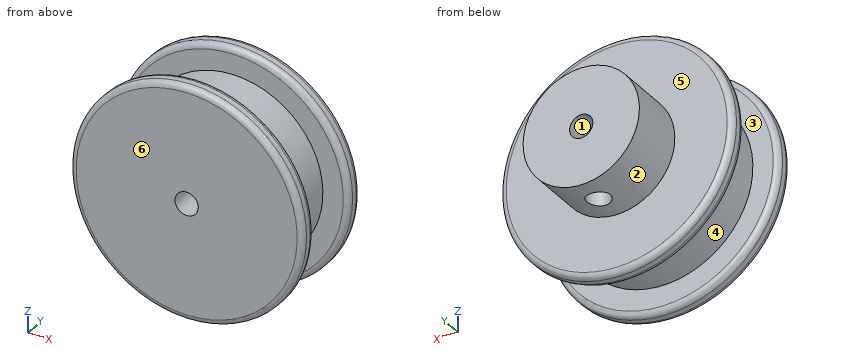
```python
from build123d import *

# Parameters (mm, degrees)
SKETCH_1_R          = 15.5
EXTRUDE_1_DEPTH     = 10
SKETCH_2_R          = 20
EXTRUDE_2_DEPTH     = 3
EXTRUDE_START       = 3
SKETCH_3_R          = 20
EXTRUDE_3_DEPTH     = 3
FILLET_2_R          = 1
SKETCH_4_R          = 2
CUT_EXTRUDE_1_DEPTH = 33.49615368
EXTRUDE_START_2     = 10
SKETCH_5_R          = 10
SKETCH_5_R_2        = 2
EXTRUDE_4_DEPTH     = 10
SKETCH_6_R          = 2
CUT_EXTRUDE_2_DEPTH = 37.455452322


with BuildPart() as part:
    # 草图1 → 凸台-拉伸1 (new body)
    with BuildSketch(Plane(origin=(0, 0, 0), x_dir=(1, 0, 0), z_dir=(0, 1, 0))):
        with Locations(Location((0, 0, 0), (0, 0, 270))):
            Circle(SKETCH_1_R)
    extrude(amount=EXTRUDE_1_DEPTH)

    # 草图2 → 凸台-拉伸2 (add)
    with BuildSketch(Plane(origin=(0, 10, 0), x_dir=(1, 0, 0), z_dir=(0, 1, 0))):
        with Locations(Location((0, 0, 0), (0, 0, 270))):
            Circle(SKETCH_2_R)
    extrude(amount=EXTRUDE_2_DEPTH)

    # 草图3 → 凸台-拉伸3 (add)
    with BuildSketch(Plane.XZ.offset(EXTRUDE_START)):
        with Locations(Location((0, 0, 0), (0, 0, 90))):
            Circle(SKETCH_3_R)
    extrude(amount=-EXTRUDE_3_DEPTH)

    # 圆角2
    fillet_2_edges = [part.edges().sort_by_distance(p)[0] for p in [
        (0, -3, -20),
        (0, 10, -20),
        (0, 13, -20),
        (0, 0, -20),
    ]]
    fillet(fillet_2_edges, radius=FILLET_2_R)

    # 草图4 → 切除-拉伸1 (cut, through all)
    with BuildSketch(Plane(origin=(0, 13, 0), x_dir=(1, 0, 0), z_dir=(0, 1, 0))):
        with Locations(Location((0, 0, 0), (0, 0, 270))):
            Circle(SKETCH_4_R)
    extrude(amount=-CUT_EXTRUDE_1_DEPTH, mode=Mode.SUBTRACT)

    # 草图5 → 凸台-拉伸4 (add)
    with BuildSketch(Plane(origin=(0, 13, 0), x_dir=(1, 0, 0), z_dir=(0, 1, 0)).offset(EXTRUDE_START_2)):
        with Locations(Location((0, 0, 0), (0, 0, 270))):
            Circle(SKETCH_5_R)
        with Locations(Location((0, 0, 0), (0, 0, 270))):
            Circle(SKETCH_5_R_2, mode=Mode.SUBTRACT)
    extrude(amount=-EXTRUDE_4_DEPTH)

    # 草图6 → 切除-拉伸2 (cut, through all)
    with BuildSketch(Plane.XY):
        with Locations((0, 18.145224443)):
            Circle(SKETCH_6_R)
    extrude(amount=-CUT_EXTRUDE_2_DEPTH, mode=Mode.SUBTRACT)


solid = part.part
```
Work out the finished part from the listing and answer in its coordinate system (mm). Face numbers are marked on the shaded views. A direction names the side the tool comes from. Coordinates: 2 decimals unless noted, no trailing zeros. Write each loop counter-clockwise with the first axis right and the second up, starting at its lowest first coordinate (ties: lowest second). Pieces come first, ordered by that corner, then holes.
Q1. Which of the six approach directions +Z, -Z, +X, -X, +Y, -Y give full straight-line access (tool end or side, diameter ignored) to the marked faces 4, 5 and 6?
Q2. Determine the mould class of the marked faces 1, 2 and 3 for opening direction Z: released by +Z, released by -Z, zero draft, split by the parting line, or undercut.
Q3. A cutting plane is placed at A-A, the plane x = 0. State how many separate pieces and enclosed holes the cut face has, then the cut area to 3 significant figures.
Q4. Each of these flat-tipped pins is pushed along its axis until it touches: pin 1 Ø4 at (y, z) = (12.5, -4) entering from -X; pin 2 Ø2.5 at (x, y) = (0, 18.15) entering from +Z; pin 3 Ø8 at (x, y) = (-5, 0) entering from -Z; pin 4 Ø3 at (x, z) = (0, 0) entering from +Y. Where does it stop, or does it pass through?
Q5. A cutting plane is placed at C-C, the plane y = 21. Give the vertices of the cut face in (x, z), then the cut area to 3 significant figures.
Q6. A cutting plane is placed at B-B, the plane y = 6.25. Give the vertices of the cut face in (x, z).
Q7. Find the intervals of material crossed by line 1 (Y direction, x = -11.5, z = -10.5); line 2 (X direction, y = 14.75, z = 0); line 3 (X direction, y = 7.75, z = 0), in increasing order.
Findings below:
1. face 4: none
1. face 5: +Y
1. face 6: +Z, -Z, +X, -X, -Y
2. face 1: undercut
2. face 2: split by the parting line
2. face 3: zero draft
3. separate pieces: 3
3. enclosed holes: 0
3. area: 612 mm2
4. pin 1: stops at x = -19.89
4. pin 2: stops at z = 10
4. pin 3: stops at z = -19.97
4. pin 4: passes through
5. outline: circle Ø20 at (0, 0); hole circle Ø4 at (0, 0)
5. area: 302 mm2
6. outline: circle Ø31 at (0, 0); hole circle Ø4 at (0, 0)
7. line 1: y = -3 to 0, 10 to 13
7. line 2: x = -10 to -2, 2 to 10
7. line 3: x = -15.5 to -2, 2 to 15.5
